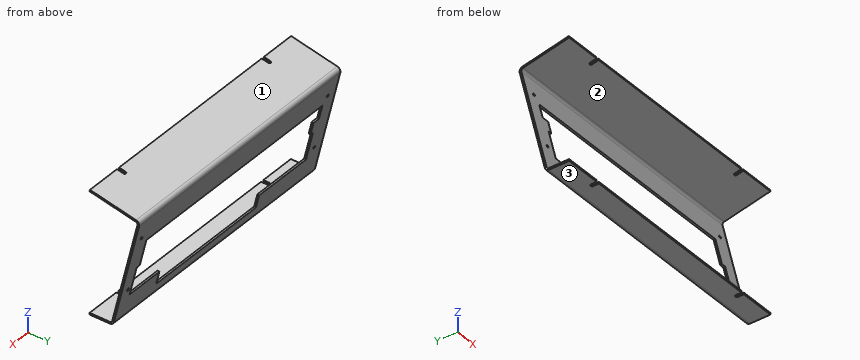
```python
from build123d import *

# Parameters (mm, degrees)
BASE_FLANGE1_DEPTH = 348
CUT_EXTRUDE1_REACH = 391.047
SKETCH6_R          = 1.95
CUT_EXTRUDE2_REACH = 384.238
SKETCH7_R          = 1.95
CUT_EXTRUDE3_REACH = 389.236
CUT_EXTRUDE4_REACH = 389.217
SKETCH9_R          = 1.75


# Sheet-metal steps are written as plain solids
with BuildPart() as part:
    # Sketch1 → Base-Flange1 (new body)
    with BuildSketch(Plane(origin=(0, 0, 0), x_dir=(0, 0, -1), z_dir=(1, 0, 0))):
        with BuildLine():
            Line((-156.66, 0), (-143.903368262, 60.704710735))
            ThreePointArc((-143.903368262, 60.704710735), (-142.570157767, 62.623791445), (-140.264606132, 63.004255181))
            Line((-140.264606132, 63.004255181), (-2.297114265, 29.753612482))
            ThreePointArc((-2.297114265, 29.753612482), (-0.643237686, 28.693367991), (0, 26.837116015))
            Line((0, 26.837116015), (0, 0))
            Line((0, 0), (2.286, 0))
            Line((2.286, 0), (2.286, 26.837116015))
            ThreePointArc((2.286, 26.837116015), (1.152615197, 30.107831996), (-1.761515334, 31.97598279))
            Line((-1.761515334, 31.97598279), (-139.729007202, 65.226625489))
            ThreePointArc((-139.729007202, 65.226625489), (-143.791389182, 64.556248387), (-146.140506074, 61.174828176))
            Line((-146.140506074, 61.174828176), (-158.897137813, 0.47011744))
            Line((-158.897137813, 0.47011744), (-156.66, 0))
        make_face()
    extrude(amount=BASE_FLANGE1_DEPTH)

    # Sketch6 → Cut-Extrude1 (cut, up to next)
    with BuildSketch(Plane(origin=(0, 0, -2.286), x_dir=(-1, 0, 0), z_dir=(0, 0, -1)), mode=Mode.PRIVATE) as cut_extrude1_sk1:
        with BuildLine():
            Line((-51.45, 7.64), (-51.45, 0))
            Line((-51.45, 0), (-47.55, 0))
            Line((-47.55, 0), (-47.55, 7.64))
            ThreePointArc((-47.55, 7.64), (-49.5, 5.69), (-51.45, 7.64))
        make_face()
    cut_extrude1_tool1 = extrude(cut_extrude1_sk1.sketch, amount=-CUT_EXTRUDE1_REACH, mode=Mode.PRIVATE) & part.part
    # Sketch6 → Cut-Extrude1 (cut, up to next)
    with BuildSketch(Plane(origin=(0, 0, -2.286), x_dir=(-1, 0, 0), z_dir=(0, 0, -1)), mode=Mode.PRIVATE) as cut_extrude1_sk2:
        with Locations((-49.5, 7.64)):
            Circle(SKETCH6_R)
    cut_extrude1_tool2 = extrude(cut_extrude1_sk2.sketch, amount=-CUT_EXTRUDE1_REACH, mode=Mode.PRIVATE) & part.part
    # Sketch6 → Cut-Extrude1 (cut, up to next)
    with BuildSketch(Plane(origin=(0, 0, -2.286), x_dir=(-1, 0, 0), z_dir=(0, 0, -1)), mode=Mode.PRIVATE) as cut_extrude1_sk3:
        with BuildLine():
            ThreePointArc((-298.13, 7.64), (-300.08, 5.69), (-302.03, 7.64))
            Line((-302.03, 7.64), (-302.03, 0))
            Line((-302.03, 0), (-298.13, 0))
            Line((-298.13, 0), (-298.13, 7.64))
        make_face()
    cut_extrude1_tool3 = extrude(cut_extrude1_sk3.sketch, amount=-CUT_EXTRUDE1_REACH, mode=Mode.PRIVATE) & part.part
    # Sketch6 → Cut-Extrude1 (cut, up to next)
    with BuildSketch(Plane(origin=(0, 0, -2.286), x_dir=(-1, 0, 0), z_dir=(0, 0, -1)), mode=Mode.PRIVATE) as cut_extrude1_sk4:
        with Locations((-300.08, 7.64)):
            Circle(SKETCH6_R)
    cut_extrude1_tool4 = extrude(cut_extrude1_sk4.sketch, amount=-CUT_EXTRUDE1_REACH, mode=Mode.PRIVATE) & part.part
    add(cut_extrude1_tool1.solids().sort_by_distance((49.5, 3.069742, -2.286))[0], mode=Mode.SUBTRACT)
    add(cut_extrude1_tool2.solids().sort_by_distance((49.5, 7.64, -2.286))[0], mode=Mode.SUBTRACT)
    add(cut_extrude1_tool3.solids().sort_by_distance((300.08, 3.069742, -2.286))[0], mode=Mode.SUBTRACT)
    add(cut_extrude1_tool4.solids().sort_by_distance((300.08, 7.64, -2.286))[0], mode=Mode.SUBTRACT)

    # Sketch7 → Cut-Extrude2 (cut, up to next)
    with BuildSketch(Plane(origin=(0, 31.998723581, 152.271641819), x_dir=(1, 0, 0), z_dir=(0, 0.20565067377814067, 0.9786254648100042)), mode=Mode.PRIVATE) as cut_extrude2_sk1:
        with Locations((299.45, -23.507234554)):
            Circle(SKETCH7_R)
    cut_extrude2_tool1 = extrude(cut_extrude2_sk1.sketch, amount=-CUT_EXTRUDE2_REACH, mode=Mode.PRIVATE) & part.part
    # Sketch7 → Cut-Extrude2 (cut, up to next)
    with BuildSketch(Plane(origin=(0, 31.998723581, 152.271641819), x_dir=(1, 0, 0), z_dir=(0, 0.20565067377814067, 0.9786254648100042)), mode=Mode.PRIVATE) as cut_extrude2_sk2:
        with BuildLine():
            Line((297.5, -23.507234554), (297.5, -32.217234554))
            Line((297.5, -32.217234554), (301.4, -32.217234554))
            Line((301.4, -32.217234554), (301.4, -23.507234554))
            ThreePointArc((301.4, -23.507234554), (299.45, -25.457234554), (297.5, -23.507234554))
        make_face()
    cut_extrude2_tool2 = extrude(cut_extrude2_sk2.sketch, amount=-CUT_EXTRUDE2_REACH, mode=Mode.PRIVATE) & part.part
    # Sketch7 → Cut-Extrude2 (cut, up to next)
    with BuildSketch(Plane(origin=(0, 31.998723581, 152.271641819), x_dir=(1, 0, 0), z_dir=(0, 0.20565067377814067, 0.9786254648100042)), mode=Mode.PRIVATE) as cut_extrude2_sk3:
        with Locations((49.06, -23.507234554)):
            Circle(SKETCH7_R)
    cut_extrude2_tool3 = extrude(cut_extrude2_sk3.sketch, amount=-CUT_EXTRUDE2_REACH, mode=Mode.PRIVATE) & part.part
    # Sketch7 → Cut-Extrude2 (cut, up to next)
    with BuildSketch(Plane(origin=(0, 31.998723581, 152.271641819), x_dir=(1, 0, 0), z_dir=(0, 0.20565067377814067, 0.9786254648100042)), mode=Mode.PRIVATE) as cut_extrude2_sk4:
        with BuildLine():
            ThreePointArc((51.01, -23.507234554), (49.06, -25.457234554), (47.11, -23.507234554))
            Line((47.11, -23.507234554), (47.11, -32.217234554))
            Line((47.11, -32.217234554), (51.01, -32.217234554))
            Line((51.01, -32.217234554), (51.01, -23.507234554))
        make_face()
    cut_extrude2_tool4 = extrude(cut_extrude2_sk4.sketch, amount=-CUT_EXTRUDE2_REACH, mode=Mode.PRIVATE) & part.part
    add(cut_extrude2_tool1.solids().sort_by_distance((299.45, 8.993945, 157.10592))[0], mode=Mode.SUBTRACT)
    add(cut_extrude2_tool2.solids().sort_by_distance((299.45, 3.995548, 158.156295))[0], mode=Mode.SUBTRACT)
    add(cut_extrude2_tool3.solids().sort_by_distance((49.06, 8.993945, 157.10592))[0], mode=Mode.SUBTRACT)
    add(cut_extrude2_tool4.solids().sort_by_distance((49.06, 3.995548, 158.156295))[0], mode=Mode.SUBTRACT)

    # Sketch8 → Cut-Extrude3 (cut, up to next)
    with BuildSketch(Plane(origin=(0, 29.819457861, -7.186592475), x_dir=(1, 0, 0), z_dir=(0, 0.9721654890653966, -0.23429524508670335)), mode=Mode.PRIVATE) as cut_extrude3_sk1:
        Polygon((324.49, -115.414305141), (19.74, -115.414305141), (19.74, -95.714305141), (29.26, -95.714305141), (29.26, -78.184305141), (24.81, -78.184305141), (24.81, -38.504305141), (105.77, -38.504305141), (105.77, -20.504305141), (278.31, -20.504305141), (278.31, -38.504305141), (329.83, -38.504305141), (329.83, -78.184305141), (324.49, -78.184305141), align=None)
    cut_extrude3_tool1 = extrude(cut_extrude3_sk1.sketch, amount=-CUT_EXTRUDE3_REACH, mode=Mode.PRIVATE) & part.part
    add(cut_extrude3_tool1.solids().sort_by_distance((177.78099, 46.525494, 62.132065))[0], mode=Mode.SUBTRACT)

    # Sketch9 → Cut-Extrude4 (cut, up to next)
    with BuildSketch(Plane(origin=(0, 27.597087553, -6.650993545), x_dir=(1, 0, 0), z_dir=(0, -0.9721654890653966, 0.23429524508670332)), mode=Mode.PRIVATE) as cut_extrude4_sk1:
        with Locations(Location((13.84, 125.740713464, 0), (0, 0, 270))):
            Circle(SKETCH9_R)
    cut_extrude4_tool1 = extrude(cut_extrude4_sk1.sketch, amount=-CUT_EXTRUDE4_REACH, mode=Mode.PRIVATE) & part.part
    # Sketch9 → Cut-Extrude4 (cut, up to next)
    with BuildSketch(Plane(origin=(0, 27.597087553, -6.650993545), x_dir=(1, 0, 0), z_dir=(0, -0.9721654890653966, 0.23429524508670332)), mode=Mode.PRIVATE) as cut_extrude4_sk2:
        with Locations(Location((335.82, 125.740713464, 0), (0, 0, 270))):
            Circle(SKETCH9_R)
    cut_extrude4_tool2 = extrude(cut_extrude4_sk2.sketch, amount=-CUT_EXTRUDE4_REACH, mode=Mode.PRIVATE) & part.part
    # Sketch9 → Cut-Extrude4 (cut, up to next)
    with BuildSketch(Plane(origin=(0, 27.597087553, -6.650993545), x_dir=(1, 0, 0), z_dir=(0, -0.9721654890653966, 0.23429524508670332)), mode=Mode.PRIVATE) as cut_extrude4_sk3:
        with Locations(Location((335.82, 49.560713464, 0), (0, 0, 270))):
            Circle(SKETCH9_R)
    cut_extrude4_tool3 = extrude(cut_extrude4_sk3.sketch, amount=-CUT_EXTRUDE4_REACH, mode=Mode.PRIVATE) & part.part
    # Sketch9 → Cut-Extrude4 (cut, up to next)
    with BuildSketch(Plane(origin=(0, 27.597087553, -6.650993545), x_dir=(1, 0, 0), z_dir=(0, -0.9721654890653966, 0.23429524508670332)), mode=Mode.PRIVATE) as cut_extrude4_sk4:
        with Locations(Location((13.84, 49.560713464, 0), (0, 0, 270))):
            Circle(SKETCH9_R)
    cut_extrude4_tool4 = extrude(cut_extrude4_sk4.sketch, amount=-CUT_EXTRUDE4_REACH, mode=Mode.PRIVATE) & part.part
    add(cut_extrude4_tool1.solids().sort_by_distance((13.84, 57.057539, 115.589789))[0], mode=Mode.SUBTRACT)
    add(cut_extrude4_tool2.solids().sort_by_distance((335.82, 57.057539, 115.589789))[0], mode=Mode.SUBTRACT)
    add(cut_extrude4_tool3.solids().sort_by_distance((335.82, 39.208927, 41.530222))[0], mode=Mode.SUBTRACT)
    add(cut_extrude4_tool4.solids().sort_by_distance((13.84, 39.208927, 41.530222))[0], mode=Mode.SUBTRACT)


solid = part.part
```
The listing builds one solid part. Answer for the finished solid, in the listing's coordinates (mm). Face numbers are marked on the shaded views. Give positions to 0.01 mm unless a question says otherwise; leave off trailing zeros. Order: outer loops, then holes, each group sorted by start corner. A loop starts at its lowest first (then second) coordinate and runs counter-clockwise, first axis right, second up.
Item 1: The part is cut by section C-C, the plane x = 238. Give the vertices of the cut face in (y, z), and give its area (3 significant figures).
From the geometry:
outline: (0, -2.29) - (26.84, -2.29) arc R5.29 ccw to (31.98, 1.76) - (34.62, 12.75) - (32.4, 13.28) - (29.75, 2.3) arc R3 cw to (26.84, 0) - (0, 0) - close; (0, 156.66) - (60.7, 143.9) arc R3 cw to (63, 140.26) - (54.64, 105.55) - (56.86, 105.02) - (65.23, 139.73) arc R5.29 ccw to (61.17, 146.14) - (0.47, 158.9) - close
area: 338 mm2
Item 2: Given pin 1 Ø1.5 at (x, y) = (215.5, 50.5) entering from +Z; pin 2 Ø10 at (x, z) = (312.5, 17) entering from -Y; pin 3 Ø8 at (x, y) = (265, 22.5) entering from +Z, each flat-ended and moving along its own axis, determine where each tip first touches the part or whether it passes through.
From the geometry:
pin 1: stops at z = 148.54
pin 2: stops at y = 32.09
pin 3: stops at z = 155.11
Item 3: For a pull along Z with two mould halves and no side action, classify the marked faces 1, 2 and 3 as pulls with the +Z half, pulls with the -Z half, needs draft (parallel to the pull), parting line crosses it, or undercut.
From the geometry:
face 1: pulls with the +Z half
face 2: undercut
face 3: pulls with the -Z half
Item 4: Find the intervals of material crossed by probe 1 along X at (y, z) = (34.5, 13); probe 2 along Z at (x, y) = (62.5, 4.5); probe 3 along Z at (x, y) = (333, 14), in increasing order.
From the geometry:
probe 1: x = 0 to 105.77, 278.31 to 348
probe 2: z = -2.29 to 0, 155.71 to 158.05
probe 3: z = -2.29 to 0, 153.72 to 156.05
Item 5: The part is cut by section A-A, the plane x = 84. Give the vertices of the cut face in (y, z).
From the geometry:
outline: (0, -2.29) - (26.84, -2.29) arc R5.29 ccw to (31.98, 1.76) - (38.84, 30.25) - (36.62, 30.78) - (29.75, 2.3) arc R3 cw to (26.84, 0) - (0, 0) - close; (0, 156.66) - (60.7, 143.9) arc R3 cw to (63, 140.26) - (54.64, 105.55) - (56.86, 105.02) - (65.23, 139.73) arc R5.29 ccw to (61.17, 146.14) - (0.47, 158.9) - close
Item 6: The part is cut by section B-B, the plane z = 76. Give the vertices of the cut face in (x, y).
From the geometry:
outline: (0, 47.52) - (29.26, 47.52) - (29.26, 49.87) - (0, 49.87) - close; (324.49, 47.52) - (348, 47.52) - (348, 49.87) - (324.49, 49.87) - close
